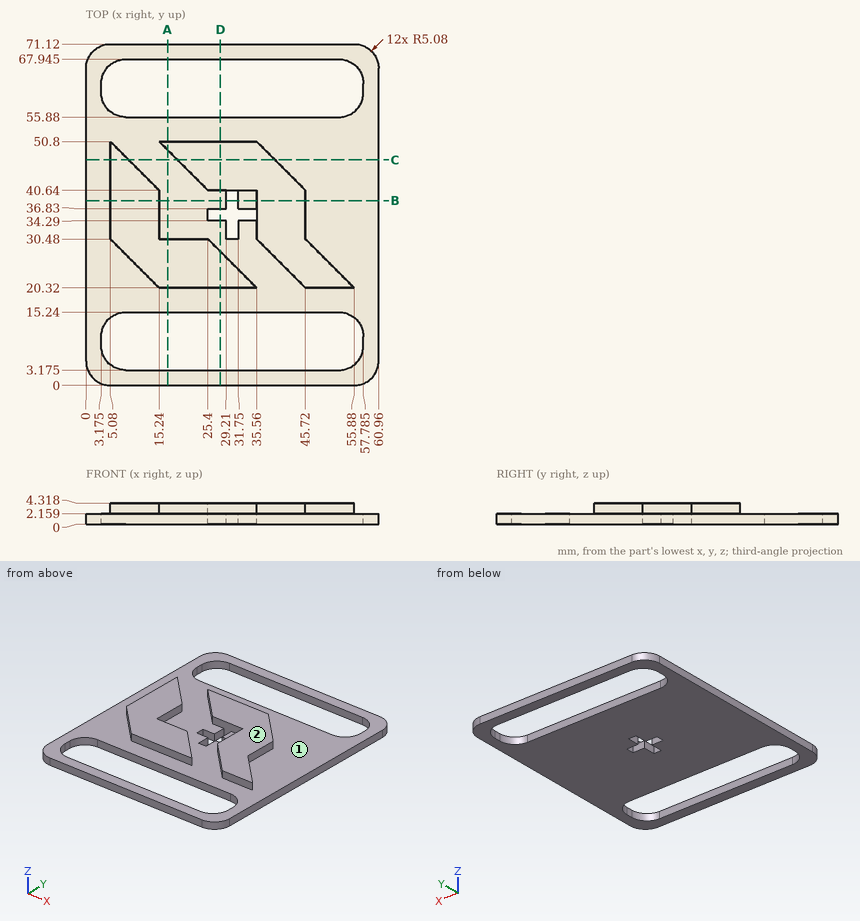
Can you work these out from the drawing? Everything is in mm from the part's minimum corner. Round coordinates to 2 decimals unless told otherwise and drop trailing zeros. Order: outer loops, then holes, each group sorted by start corner. A loop starts at its lowest first (then second) coordinate and runs counter-clockwise, first axis right, second up.
(1) I'm going to push flat-ended pins straight in: pin 1 (0.6 mm diameter, centred on y = 34, z = 3, fed in from +X); pin 2 (1.3 mm diameter, centred on x = 28.5, z = 3, fed in from -Y); pin 3 (12 mm diameter, centred on x = 25.5, y = 10.5, fed in from +Z). Where does each tip first touch, or does it pass through?
Results are:
pin 1: stops at x = 45.72
pin 2: stops at y = 20.32
pin 3: stops at z = 2.16
(2) If I drill on L1, parallel to Y at x = 15.5, z = 1.65 (3 decimals); L2, parallel to Y at x = 34, z = 1.9 (3 decimals); L3, parallel to X at y = 36.5, z = 1.1, over which ranges is the centre line in solid material (lowest first)?
Results are:
L1: y = 0 to 3.175, 15.24 to 55.88, 67.945 to 71.12
L2: y = 0 to 3.175, 15.24 to 34.29, 36.83 to 55.88, 67.945 to 71.12
L3: x = 0 to 25.4, 35.56 to 60.96
(3) We'd pull the mould along X, two halves only. Please class the marked faces 1 and 2: +X half, -X half, draft (parallel to the pull), parting line (faces both ways), or undercut.
Results are:
face 1: undercut
face 2: draft
(4) If we section it at A-A (x = 17): Please give me the cut outline in (y, z) (3 decimals), plus the area to 3 significant figures.
Results are:
outline: (0, 0) - (3.175, 0) - (3.175, 2.159) - (0, 2.159) - close; (15.24, 0) - (55.88, 0) - (55.88, 2.159) - (50.8, 2.159) - (50.8, 4.318) - (49.04, 4.318) - (49.04, 2.159) - (30.48, 2.159) - (30.48, 4.318) - (20.32, 4.318) - (20.32, 2.159) - (15.24, 2.159) - close; (67.945, 0) - (71.12, 0) - (71.12, 2.159) - (67.945, 2.159) - close
area: 127 mm2
(5) If we section it at D-D (x = 28): Please give me the cut outline in (y, z) (3 decimals).
Results are:
outline: (0, 0) - (3.175, 0) - (3.175, 2.159) - (0, 2.159) - close; (15.24, 0) - (34.29, 0) - (34.29, 2.159) - (27.88, 2.159) - (27.88, 4.318) - (20.32, 4.318) - (20.32, 2.159) - (15.24, 2.159) - close; (36.83, 0) - (55.88, 0) - (55.88, 2.159) - (50.8, 2.159) - (50.8, 4.318) - (40.64, 4.318) - (40.64, 2.159) - (36.83, 2.159) - close; (67.945, 0) - (71.12, 0) - (71.12, 2.159) - (67.945, 2.159) - close
(6) If we section it at B-B (y = 38.5): Please give me the cut outline in (x, z).
Results are:
outline: (0, 0) - (29.21, 0) - (29.21, 2.16) - (15.24, 2.16) - (15.24, 4.32) - (5.08, 4.32) - (5.08, 2.16) - (0, 2.16) - close; (31.75, 0) - (60.96, 0) - (60.96, 2.16) - (45.72, 2.16) - (45.72, 4.32) - (35.56, 4.32) - (35.56, 2.16) - (31.75, 2.16) - close
(7) If we section it at C-C (y = 47): Please give me the cut outline in (x, z).
Results are:
outline: (0, 0) - (60.96, 0) - (60.96, 2.16) - (39.36, 2.16) - (39.36, 4.32) - (19.04, 4.32) - (19.04, 2.16) - (8.88, 2.16) - (8.88, 4.32) - (5.08, 4.32) - (5.08, 2.16) - (0, 2.16) - close
